Can you work these out from the model? Positions are in its coordinate system, mm. Face numbers are marked on the shaded views. Coordinates: 2 decimals unless noted, no trailing zeros. Write each loop counter-clockwise with the first axis right and the second up, starting at its lowest first coordinate (ties: lowest second). Pieces come first, ordered by that corner, then holes. Notation, with made-up numbers: M -24.75,43.25 L -16.75,43.25 A19 ccw -16.75,73.25 Z; hole C 0.25,-6 d11. An arc over 180 degrees is marked long. Answer as a JSON object with one key per item and string values. Group by question number.
from build123d import *

# Parameters (mm, degrees)
SKETCH_W      = 63.5
SKETCH_H      = 44.45
PAD_DEPTH     = 1.27
SKETCH001_W   = 60.452
SKETCH001_H   = 41.402
SKETCH001_W_2 = 58.42
SKETCH001_H_2 = 39.37
PAD001_DEPTH  = 3.81
SKETCH002_R   = 2.794
POCKET_DEPTH  = 5.081
SKETCH003_R   = 3.81
SKETCH003_R_2 = 2.794
PAD002_DEPTH  = 5.08


with BuildPart() as part:
    # Sketch → Pad (new body)
    with BuildSketch(Plane.XY):
        with Locations((31.75, 22.225)):
            Rectangle(SKETCH_W, SKETCH_H)
    extrude(amount=PAD_DEPTH)

    # Sketch001 (on Face5 of Pad) → Pad001 (join)
    with BuildSketch(Plane(origin=(0, 0, 0), x_dir=(1, 0, 0), z_dir=(0, 0, -1))):
        with Locations((31.75, -22.225)):
            Rectangle(SKETCH001_W, SKETCH001_H)
        with Locations((31.75, -22.225)):
            Rectangle(SKETCH001_W_2, SKETCH001_H_2, mode=Mode.SUBTRACT)
    extrude(amount=PAD001_DEPTH)

    # Sketch002 (on Face5 of Pad001) → Pocket (cut, through all)
    with BuildSketch(Plane.XY.offset(1.27)):
        with Locations((33.02, 30.48)):
            Circle(SKETCH002_R)
        with BuildLine():
            ThreePointArc((54.61, 5.08), (58.42, 8.89), (54.61, 12.7))
            Line((54.61, 12.7), (35.56, 12.7))
            ThreePointArc((35.56, 12.7), (31.75, 8.89), (35.56, 5.08))
            Line((54.61, 5.08), (35.56, 5.08))
        make_face()
    extrude(amount=-POCKET_DEPTH, mode=Mode.SUBTRACT)

    # Sketch003 (on Face17 of Pocket) → Pad002 (join)
    with BuildSketch(Plane(origin=(0, 0, 0), x_dir=(1, 0, 0), z_dir=(0, 0, -1))):
        with Locations((33.02, -30.48)):
            Circle(SKETCH003_R)
        with Locations((33.02, -30.48)):
            Circle(SKETCH003_R_2, mode=Mode.SUBTRACT)
    extrude(amount=PAD002_DEPTH)


solid = part.part
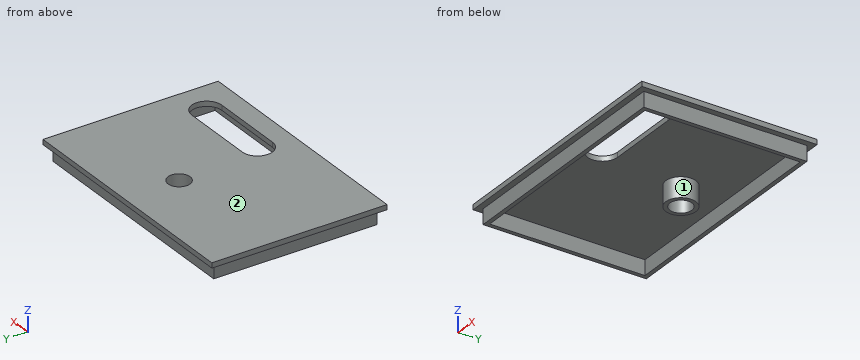
Q1. Will these pins go through, and if not, where does the flat tip stop? pin 1 (10 mm diameter, centred on x = 16.5, y = 14, fed in from -Z); pin 2 (1.5 mm diameter, centred on x = 31.5, z = -1.5, fed in from -Y); pin 3 (1.9 mm diameter, centred on y = 19, z = -1.5, fed in from +X); pin 4 (12.5 mm diameter, centred on x = 31, y = 21, fed in from -Z).
Q2. If we section it at A-A on y = 30.48: List the corners of the cut face in (x, z) for me, and give its area (3 significant figures).
Q3. If we section it at B-B on z = -1: List the corners of the cut face in (x, y) for me, and give its area (3 significant figures).
Q4. We'd pull the mould along Y, two halves only. Please class the marked faces 1 and 2: pulls with the +Y half, pulls with the -Y half, needs draft (parallel to the pull), parting line crosses it, or undercut.
Q5. Please list where these lines run through material, in increasing order: L1, parallel to Y at x = 33.02, z = -3; L2, parallel to X at y = 30.48, z = -0.5; L3, parallel to Y at x = 12.5, z = -0.5.
Q6. If we section it at C-C on x = 33.02: List the corners of the cut face in (y, z) for me.
Q7. If we section it at D-D on y = 8.89: List the corners of the cut face in (x, z) for me.
Reply:
{
 "1": {"pin 1": "z = 0", "pin 2": "y = 1.52", "pin 3": "x = 61.98", "pin 4": "z = -5.08"},
 "2": {"outline": "M 0,0 L 1.52,0 L 1.52,-3.81 L 2.54,-3.81 L 2.54,0 L 29.21,0 L 29.21,-5.08 L 30.23,-5.08 L 30.23,1.27 L 0,1.27 Z; M 35.81,-5.08 L 36.83,-5.08 L 36.83,0 L 60.96,0 L 60.96,-3.81 L 61.98,-3.81 L 61.98,0 L 63.5,0 L 63.5,1.27 L 35.81,1.27 Z", "area": "91.6 mm^2"},
 "3": {"outline": "M 1.52,1.52 L 61.98,1.52 L 61.98,42.93 L 1.52,42.93 Z; C 33.02,30.48 d7.62; hole M 2.54,2.54 L 60.96,2.54 L 60.96,41.91 L 2.54,41.91 Z; hole C 33.02,30.48 d5.59", "area": "224 mm^2"},
 "4": {"face 1": "undercut", "face 2": "needs draft"},
 "5": {"L1": "1.52 to 2.54, 26.67 to 27.69, 33.27 to 34.29, 41.91 to 42.93", "L2": "1.52 to 2.54, 29.21 to 30.23, 35.81 to 36.83, 60.96 to 61.98", "L3": "1.52 to 2.54, 41.91 to 42.93"},
 "6": {"outline": "M 0,0 L 1.52,0 L 1.52,-3.81 L 2.54,-3.81 L 2.54,0 L 6.05,0 L 6.05,1.27 L 0,1.27 Z; M 11.73,0 L 26.67,0 L 26.67,-5.08 L 27.69,-5.08 L 27.69,1.27 L 11.73,1.27 Z; M 33.27,-5.08 L 34.29,-5.08 L 34.29,0 L 41.91,0 L 41.91,-3.81 L 42.93,-3.81 L 42.93,0 L 44.45,0 L 44.45,1.27 L 33.27,1.27 Z"},
 "7": {"outline": "M 0,0 L 1.52,0 L 1.52,-3.81 L 2.54,-3.81 L 2.54,0 L 31.75,0 L 31.75,1.27 L 0,1.27 Z; M 58.42,0 L 60.96,0 L 60.96,-3.81 L 61.98,-3.81 L 61.98,0 L 63.5,0 L 63.5,1.27 L 58.42,1.27 Z"}
}
